from build123d import *

# Parameters (mm, degrees)
SKETCH1_R           = 30
BOSS_EXTRUDE1_DEPTH = 100
SKETCH2_R           = 20.5
CUT_EXTRUDE1_DEPTH  = 150
SKETCH3_R           = 3.175
BOSS_EXTRUDE3_DEPTH = 10
CUT_EXTRUDE2_REACH  = 144.215
SKETCH4_W           = 10
SKETCH4_H           = 20


with BuildPart() as part:
    # Sketch1 → Boss-Extrude1 (new, symmetric)
    with BuildSketch(Plane(origin=(0, 0, 0), x_dir=(1, 0, 0), z_dir=(0, 1, 0))):
        with Locations(Location((0, 0, 0), (0, 0, 270))):
            Circle(SKETCH1_R)
    extrude(amount=BOSS_EXTRUDE1_DEPTH, both=True)

    # Sketch2 → Cut-Extrude1 (cut)
    with BuildSketch(Plane(origin=(0, 100, 0), x_dir=(1, 0, 0), z_dir=(0, 1, 0))):
        with Locations(Location((0, 0, 0), (0, 0, 270))):
            Circle(SKETCH2_R)
    extrude(amount=-CUT_EXTRUDE1_DEPTH, mode=Mode.SUBTRACT)

    # Sketch3 → Boss-Extrude3 (add, symmetric)
    with BuildSketch(Plane(origin=(0, 0, 0), x_dir=(0, 0, -1), z_dir=(1, 0, 0))):
        Polygon((20.5, 100), (35, 100), (35, 110), (55, 110), (55, 80), (20.5, 80), align=None)
        with Locations((45, 100)):
            Circle(SKETCH3_R, mode=Mode.SUBTRACT)
    boss_extrude3 = extrude(amount=BOSS_EXTRUDE3_DEPTH, both=True)

    # Cut-Extrude2: up to this face of the body (flat: up to its plane)
    cut_extrude2_end = Plane(part.part.faces().sort_by_distance((0, 105, -35))[0])
    # Sketch4 → Cut-Extrude2 (cut, up to the picked face)
    with BuildSketch(Plane(origin=(0, 0, -55), x_dir=(-1, 0, 0), z_dir=(0, 0, -1)), mode=Mode.PRIVATE) as cut_extrude2_sk1:
        with Locations((0, 100)):
            Rectangle(SKETCH4_W, SKETCH4_H)
    cut_extrude2_tool1 = split(extrude(cut_extrude2_sk1.sketch, amount=-CUT_EXTRUDE2_REACH, mode=Mode.PRIVATE), bisect_by=cut_extrude2_end, keep=Keep.BOTH, mode=Mode.PRIVATE)
    cut_extrude2 = cut_extrude2_tool1.solids().sort_by(Axis((0, 100, -55), (0, 0, 1)))[0]
    add(cut_extrude2, mode=Mode.SUBTRACT)

    # Mirror1: Boss-Extrude3, Cut-Extrude2 across plane
    add(boss_extrude3.mirror(Plane.XY))
    add(cut_extrude2.mirror(Plane.XY), mode=Mode.SUBTRACT)


solid = part.part
Here's how the part is built. I have some questions about the finished solid (model axes, mm). A direction names the side the tool comes from. Coordinates: 2 decimals unless noted, no trailing zeros. Loops run counter-clockwise (first coordinate to the right, second up) from the corner with the lowest first, then second, coordinate; pieces in that order, holes last.
1. Imagine slicing it at A-A, the plane z = -45. Please give me the cut outline in (x, y) (3 decimals), and give its area (4 significant figures).
2. I need wall thicknesses on L1, parallel to X at y = 2, z = 0; L2, parallel to Y at x = 8.5, z = 45 (3 decimals). Which ranges of each line are inside material? Lowest first, please.
3. If we mould it in two halves opening along Z, with no side actions, what happens to faces 1 (the cylindrical face through (-7.535, 102.677, -46.707)), 2 (the flat face through (0, 90, -45)), 3 (the flat face through (0, 89, 55))? For each: pulls with the +Z half, pulls with the -Z half, needs draft (parallel to the pull), parting line crosses it, or undercut.
4. Imagine slicing it at D-D, the plane z = 0. Please give me the cut outline in (x, y), and give its area (3 significant figures).
5. For faces 4 (the flat face through (-7, 105, -35)), 5 (the flat face through (0, 95, 35)), 6 (the flat face through (-5, 97.6, -47.4)), 7 (the cylindrical face through (-20.013, 26.05, -4.444)), 8 (the flat face through (10, 95, 42)), which set-ups out of +Z, -Z, +X, -X, +Y, -Y let a thin tool reach every point of the face, with its end or its side?
6. For P1, Ø8, axis at x = -15.5, z = 13, coming from the +Y side; P2, Ø1.5, axis at y = 33, z = -18, coming from the -X side; P3, Ø5.5, axis at y = 100, z = -45, coming from the -X side; P4, Ø8, axis at y = 97.5, z = -45, coming from the -X side, each with a flat end and sliding along its axis, tell me the tip position at first contact or that it passes through.
7. Imagine slicing it at B-B, the plane y = 21. Please give me the cut outline in (x, z), and give its area (3 significant figures).
8. Imagine slicing it at C-C, the plane x = 0. Please give me the cut outline in (y, z), and give its area (3 significant figures).
Taken from the geometry:
1. outline: (-10, 80) - (10, 80) - (10, 96.825) - (5, 96.825) - (5, 90) - (-5, 90) - (-5, 96.825) - (-10, 96.825) - close; (-10, 103.175) - (-5, 103.175) - (-5, 110) - (-10, 110) - close; (5, 103.175) - (10, 103.175) - (10, 110) - (5, 110) - close
1. area: 336.5 mm2
2. L1: x = -30 to -20.5, 20.5 to 30
2. L2: y = 80 to 96.825, 103.175 to 110
3. face 1: undercut
3. face 2: needs draft
3. face 3: pulls with the +Z half
4. outline: (-30, -100) - (30, -100) - (30, 100) - (20.5, 100) - (20.5, -50) - (-20.5, -50) - (-20.5, 100) - (-30, 100) - close
4. area: 5,850 mm2
5. face 4: +X, -X, +Y
5. face 5: +Z, +Y
5. face 6: -Z, +Y
5. face 7: +Y
5. face 8: +Z, +X, +Y, -Y
6. P1: stops at y = 100
6. P2: stops at x = -24.54
6. P3: passes through
6. P4: stops at x = -10
7. outline: circle Ø60 at (0, 0); hole circle Ø41 at (0, 0)
7. area: 1,510 mm2
8. outline: (-100, -30) - (80, -30) - (80, -55) - (90, -55) - (90, -35) - (100, -35) - (100, -20.5) - (-50, -20.5) - (-50, 20.5) - (100, 20.5) - (100, 35) - (90, 35) - (90, 55) - (80, 55) - (80, 30) - (-100, 30) - close
8. area: 6,450 mm2
